from build123d import *

# Parameters (mm, degrees)
SKETCH1_W           = 26
SKETCH1_H           = 81
SKETCH1_W_2         = 20
SKETCH1_H_2         = 75
BOSS_EXTRUDE5_DEPTH = 16
SKETCH7_W           = 26
SKETCH7_H           = 81
BOSS_EXTRUDE6_DEPTH = 5
CUT_EXTRUDE3_DEPTH  = 3
SKETCH9_W           = 8
SKETCH9_H           = 16
CUT_EXTRUDE4_DEPTH  = 8
FILLET3_R           = 1.5


with BuildPart() as part:
    # Sketch1 → Boss-Extrude5 (new body)
    with BuildSketch(Plane.XY):
        with Locations((0.5, -22.5)):
            Rectangle(SKETCH1_W, SKETCH1_H)
        with Locations((0.5, -22.5)):
            Rectangle(SKETCH1_W_2, SKETCH1_H_2, mode=Mode.SUBTRACT)
    extrude(amount=BOSS_EXTRUDE5_DEPTH)

    # Sketch7 → Boss-Extrude6 (add)
    with BuildSketch(Plane.XY.offset(16)):
        with Locations((0.5, -22.5)):
            Rectangle(SKETCH7_W, SKETCH7_H)
        with BuildLine():
            Line((2.05, 11.5), (2.05, 3.5))
            ThreePointArc((2.05, 3.5), (0.5, 1.95), (-1.05, 3.5))
            Line((-1.05, 3.5), (-1.05, 11.5))
            ThreePointArc((-1.05, 11.5), (0.5, 13.05), (2.05, 11.5))
        make_face(mode=Mode.SUBTRACT)
        with BuildLine():
            Line((2.05, -56.5), (2.05, -48.5))
            ThreePointArc((2.05, -48.5), (0.5, -46.95), (-1.05, -48.5))
            Line((-1.05, -48.5), (-1.05, -56.5))
            ThreePointArc((-1.05, -56.5), (0.5, -58.05), (2.05, -56.5))
        make_face(mode=Mode.SUBTRACT)
    extrude(amount=BOSS_EXTRUDE6_DEPTH)

    # Sketch8 → Cut-Extrude3 (cut)
    with BuildSketch(Plane(origin=(0, 0, 16), x_dir=(-1, 0, 0), z_dir=(0, 0, -1))):
        with BuildLine():
            Line((2.75, 11.5), (2.75, 3.5))
            ThreePointArc((2.75, 3.5), (-0.5, 0.25), (-3.75, 3.5))
            Line((-3.75, 3.5), (-3.75, 11.5))
            ThreePointArc((-3.75, 11.5), (-0.5, 14.75), (2.75, 11.5))
        make_face()
        with BuildLine():
            Line((2.75, -56.5), (2.75, -48.5))
            ThreePointArc((2.75, -48.5), (-0.5, -45.25), (-3.75, -48.5))
            Line((-3.75, -48.5), (-3.75, -56.5))
            ThreePointArc((-3.75, -56.5), (-0.5, -59.75), (2.75, -56.5))
        make_face()
    extrude(amount=-CUT_EXTRUDE3_DEPTH, mode=Mode.SUBTRACT)

    # Sketch9 → Cut-Extrude4 (cut)
    with BuildSketch(Plane(origin=(0, 18, 0), x_dir=(1, 0, 0), z_dir=(0, 1, 0))):
        with Locations((9.5, -8)):
            Rectangle(SKETCH9_W, SKETCH9_H)
    extrude(amount=-CUT_EXTRUDE4_DEPTH, mode=Mode.SUBTRACT)

    # Fillet3
    fillet3_edges = [part.edges().sort_by_distance(p)[0] for p in [
        (-12.5, -63, 10.5),
        (0.5, -63, 21),
        (13.5, -63, 10.5),
        (13.5, -22.5, 21),
        (9.5, 18, 16),
        (13.5, 14, 16),
        (-12.5, -22.5, 21),
        (10.5, 10, 8),
        (5.5, 15, 8),
        (5.5, 18, 8),
        (13.5, 10, 8),
        (13.5, 18, 18.5),
        (-12.5, 18, 10.5),
        (0.5, 18, 21),
    ]]
    fillet(fillet3_edges, radius=FILLET3_R - 0.0001)  # a hair under: the kernel refuses the full size


solid = part.part
Design review of the part built by this model. Coordinates are the model's own, in mm. A direction names the side the tool comes from. Give positions to 0.01 mm unless a question says otherwise; leave off trailing zeros. Order: outer loops, then holes, each group sorted by start corner. A loop starts at its lowest first (then second) coordinate and runs counter-clockwise, first axis right, second up.
1. Add section A-A, the plane x = 0.5. State the section outline as (y, z) points.
Solution:
outline: (-63, 0) - (-60, 0) - (-60, 16) - (-59.75, 16) - (-59.75, 19) - (-58.05, 19) - (-58.05, 21) - (-61.5, 21) arc R1.5 ccw to (-63, 19.5) - close; (-46.95, 19) - (-45.25, 19) - (-45.25, 16) - (0.25, 16) - (0.25, 19) - (1.95, 19) - (1.95, 21) - (-46.95, 21) - close; (13.05, 19) - (14.75, 19) - (14.75, 16) - (15, 16) - (15, 0) - (18, 0) - (18, 19.5) arc R1.5 ccw to (16.5, 21) - (13.05, 21) - close
2. Add section C-C, the plane z = 18.25. State the section outline as (x, y) points, then the cut area to 3 significant figures.
Solution:
outline: (-12.5, -61.5) arc R1.5 ccw to (-11, -63) - (12, -63) arc R1.5 ccw to (13.5, -61.5) - (13.5, 16.5) arc R1.5 ccw to (12, 18) - (-11, 18) arc R1.5 ccw to (-12.5, 16.5) - close; hole (-2.75, -56.5) arc R3.25 ccw to (3.75, -56.5) - (3.75, -48.5) arc R3.25 ccw to (-2.75, -48.5) - close; hole (-2.75, 3.5) arc R3.25 ccw to (3.75, 3.5) - (3.75, 11.5) arc R3.25 ccw to (-2.75, 11.5) - close
area: 1,930 mm2
3. Mouldability with a two-part tool opening along Y and no side actions: class faces 6 (the flat face through (0, -60, 8)), 7 (the flat face through (-10, -28, 0)), 8 (the flat face through (-2, 18, 10)), 9 (the flat face through (2.05, 8, 20)) as +Y half, -Y half, draft (parallel to the pull), parting line (faces both ways), or undercut.
Solution:
face 6: undercut
face 7: draft
face 8: +Y half
face 9: undercut
4. For pin 1 Ø7 at (x, y) = (0.5, -50.5) entering from -Z; pin 2 Ø1 at (y, z) = (6.5, 20) entering from +X; pin 3 Ø2 at (x, z) = (10.5, 2.5) entering from +Y; pin 4 Ø3 at (x, y) = (0, 6) entering from -Z, all flat-tipped, find the tip position at first contact; note any pin that passes through.
Solution:
pin 1: stops at z = 16
pin 2: stops at x = 13.5
pin 3: stops at y = 9.91
pin 4: stops at z = 19
5. Tool access review of faces 1 (the flat face through (-12.5, -23, 10)), 2 (the cylindrical face through (0.66, 17.55, 20.57)), 3 (the cylindrical face through (0.57, 14.75, 17.48)), 4 (the cylindrical face through (5.05, 17.57, 8.63)), 5 (the flat face through (2.05, -53, 20)): name each direction out of +Z, -Z, +X, -X, +Y, -Y from which nothing blocks a thin tool from reaching the whole face with its end or side.
Solution:
face 1: +Z, -Z, -X, +Y, -Y
face 2: +Z, +X, -X, +Y
face 3: -Z
face 4: -Z, +X, +Y
face 5: +Z, -Z
6. Add section B-B, the plane y = 5. State the section outline as (x, z) points, then the cut area to 3 significant figures.
Solution:
outline: (-12.5, 0) - (-9.5, 0) - (-9.5, 16) - (-2.75, 16) - (-2.75, 19) - (-1.05, 19) - (-1.05, 21) - (-11, 21) arc R1.5 ccw to (-12.5, 19.5) - close; (2.05, 19) - (3.75, 19) - (3.75, 16) - (10.5, 16) - (10.5, 0) - (13.5, 0) - (13.5, 19.5) arc R1.5 ccw to (12, 21) - (2.05, 21) - close
area: 199 mm2
7. To check wall thickness, follow L1, parallel to Y at x = 0, z = 5.25; L2, parallel to X at y = -22, z = 5.5; L3, parallel to Z at x = -2, y = -13. State the ranges of each line that lie inside material, in increasing order.
Solution:
L1: y = -63 to -60, 15 to 18
L2: x = -12.5 to -9.5, 10.5 to 13.5
L3: z = 16 to 21
